Autodesk Inventor part; units mm, degrees
ref_plane "Work Plane1" through (0, 0, 5.3819) normal (-1, 0, 0) x (0, 0, 1)
ref_plane "YZ Plane" through (0, 0, 0) normal (1, 0, 0) x (0, 1, 0)
ref_plane "XZ Plane" through (0, 0, 0) normal (0, 1, 0) x (-1, 0, 0)
sketch "Sketch1" plane through (0, 0, 0) normal (0, 1, 0) x (-1, 0, 0)
  line L0 (8.5, 17.5) -> (-8.5, 17.5)
  line L1 (-8.5, 17.5) -> (-8.5, -17.5)
  line L2 (-8.5, -17.5) -> (8.5, -17.5)
  line L3 (8.5, -17.5) -> (8.5, 17.5)
  line L4 (8.5, 17.5) -> (-8.5, -17.5) construction
  line L5 (-8.5, 17.5) -> (8.5, -17.5) construction
  line L6 (0, -17.5) -> (0, -0.5)
  line L7 (0, -9) -> (4.75, -9) construction
  circle A0 centre (0, -9) radius 4.75 construction
  line L8 (0, 10.8819) -> (0, 5.3819) construction
  line L9 (-2.75, 10.8819) -> (-2.75, 5.3819)
  line L10 (2.75, 5.3819) -> (2.75, 10.8819)
  arc A1 (2.75, 10.8819) -> (-2.75, 10.8819) centre (0, 10.8819) ccw
  arc A2 (-2.75, 5.3819) -> (2.75, 5.3819) centre (0, 5.3819) ccw
  point P0 (0, 0)
  point P1 (0, -4.25)
  point P2 (0, -13.75)
  point P3 (-4.75, -9)
  point P4 (0, 8.1319)
  dimension "d0" = 17
  dimension "d1" = 35
  dimension "d2" = 17
  dimension "d3" = 4.75
  dimension "d4" = 2.75
  dimension "d5" = 5.5
extrude "Plate1" add sketch "Sketch1" along normal blind 3
hole "Hole1" at (0, 0, -4.25) at (0, 0, -13.75) at (-4.75, 0, -9) at (4.75, 0, -9) direction (0, 1, 0) diameter 3.2 depth 3 tip angle 118
fillet "Fillet1" radius 2 4 edges at (-8.5, 1.5, 17.5) (8.5, 1.5, 17.5) (-8.5, 1.5, -17.5) (8.5, 1.5, -17.5)
ref_plane "Work Plane1" through (0, 0, 5.3819) normal (-1, 0, 0) x (0, 0, 1)
equation "\"d12\" = Thickness"
equation "\"d6\" = Thickness"
equation "\"BendRadius\" = Thickness"
equation "\"BendReliefWidth\" = Thickness"
equation "\"BendReliefDepth\" = 0.5 * Thickness"
equation "\"CornerReliefSize\" = 4 * Thickness"
equation "\"MinimumRemnant\" = 2 * Thickness"
equation "\"TransitionRadius\" = BendRadius"
equation "\"JacobiRadiusSize\" = BendRadius"
equation "\"GapSize\" = Thickness"
properties part number "LimitSwitchMount" material "Aluminum 6061"
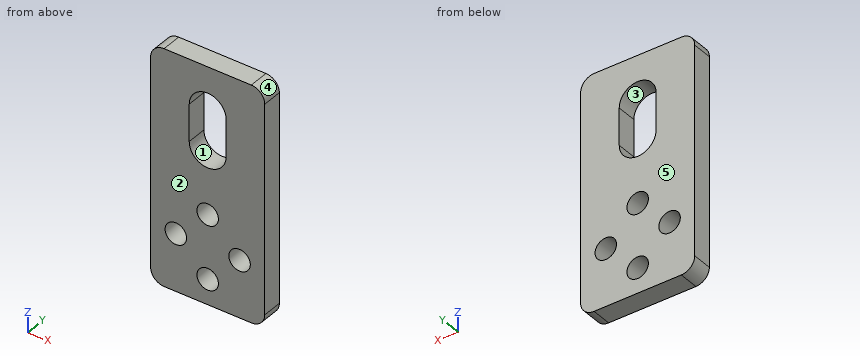
The listing builds one solid part. Answer for the finished solid, in the listing's coordinates (mm). Face numbers are marked on the shaded views. A direction names the side the tool comes from. Coordinates: 2 decimals unless noted, no trailing zeros. Write each loop counter-clockwise with the first axis right and the second up, starting at its lowest first coordinate (ties: lowest second). Pieces come first, ordered by that corner, then holes. Notation, with made-up numbers: (36.25, 17) - (76.25, 17) arc R29 ccw to (76.25, 41) - close; hole circle Ø4 at (84, 85.25). An arc over 180 degrees is marked (long way). One line per item, written item: value.
1) Find section D-D (x = 0). Give the vertices of the cut face in (y, z), and give its area (3 significant figures).
Geometry check:
outline: (0, -17.5) - (3, -17.5) - (3, -15.35) - (0, -15.35) - close; (0, -12.15) - (3, -12.15) - (3, -5.85) - (0, -5.85) - close; (0, -2.65) - (3, -2.65) - (3, 2.63) - (0, 2.63) - close; (0, 13.63) - (3, 13.63) - (3, 17.5) - (0, 17.5) - close
area: 52.8 mm2
2) Consider line 1 along Z through (x, y) = (0, 1.5); line 2 along X through (y, z) = (1.6, -9); line 3 along X through (y, z) = (1.75, -4.25). Determine where each line is inside the solid, lowest interval first. Write a range as from..to.
Geometry check:
line 1: z = -17.5..-15.35, -12.15..-5.85, -2.65..2.63, 13.63..17.5
line 2: x = -8.5..-6.35, -3.15..3.15, 6.35..8.5
line 3: x = -8.5..-1.6, 1.6..8.5
3) A tool of negligible diameter and unlimited length cuts with its end or side. For the marked faces 1 and 2, from which of +Z, -Z, +X, -X, +Y, -Y can it reach the whole face along a straight path? Write none if from no direction.
Geometry check:
face 1: +Y, -Y
face 2: +Z, -Z, +X, -X, -Y
4) Find section C-C (x = 4.75). Give the vertices of the cut face in (y, z), and give its area (3 significant figures).
Geometry check:
outline: (0, -17.5) - (3, -17.5) - (3, -10.6) - (0, -10.6) - close; (0, -7.4) - (3, -7.4) - (3, 17.5) - (0, 17.5) - close
area: 95.4 mm2
5) Find section B-B (y = 1.95). Give the vertices of the cut face in (x, z).
Geometry check:
outline: (-8.5, -15.5) arc R2 ccw to (-6.5, -17.5) - (6.5, -17.5) arc R2 ccw to (8.5, -15.5) - (8.5, 15.5) arc R2 ccw to (6.5, 17.5) - (-6.5, 17.5) arc R2 ccw to (-8.5, 15.5) - close; hole circle Ø3.2 at (-4.75, -9); hole (-2.75, 5.38) arc R2.75 ccw to (2.75, 5.38) - (2.75, 10.88) arc R2.75 ccw to (-2.75, 10.88) - close; hole circle Ø3.2 at (0, -13.75); hole circle Ø3.2 at (0, -4.25); hole circle Ø3.2 at (4.75, -9)
6) Each of these flat-tipped pins is pushed along its axis until it touches: pin 1 Ø3.5 at (x, z) = (0, -4.25) entering from -Y; pin 2 Ø3 at (x, z) = (4.75, -9) entering from +Y. Where does it stop, or does it pass through?
Geometry check:
pin 1: stops at y = 0
pin 2: passes through
7) For a pull along X with two mould halves and no side action, classify the marked faces 3, 4 and 5 as pulls with the +X half, pulls with the -X half, needs draft (parallel to the pull), parting line crosses it, or undercut.
Geometry check:
face 3: undercut
face 4: pulls with the +X half
face 5: needs draft
8) Find section A-A (z = -4.25). Give the vertices of the cut face in (x, y), and give its area (3 significant figures).
Geometry check:
outline: (-8.5, 0) - (-1.6, 0) - (-1.6, 3) - (-8.5, 3) - close; (1.6, 0) - (8.5, 0) - (8.5, 3) - (1.6, 3) - close
area: 41.4 mm2
